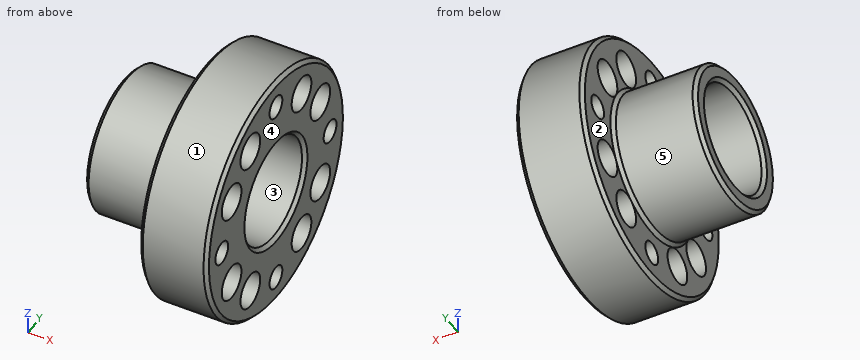
```python
from build123d import *

# Parameters (mm, degrees)
SKETCH2_R              = 3.25
CUT_EXTRUDE1_DEPTH     = 66.849562641
CHAMFER1_SIZE          = 1
SKETCH3_R              = 5
LIGHTENING_HOLES_DEPTH = 66.849562641


with BuildPart() as part:
    # Sketch1 → Revolve1 (revolve)
    with BuildSketch(Plane(origin=(0, 0, 0), x_dir=(1, 0, 0), z_dir=(0, 1, 0)), mode=Mode.PRIVATE) as revolve1_sk:
        Polygon((0, 20), (24, 20), (24, 35), (43.43, 35), (43.43, 15), (0, 15), align=None)
    revolve(revolve1_sk.sketch.rotate(Axis((0, 0, 0), (1, 0, 0)), 180), axis=Axis((0, 0, 0), (1, 0, 0)))

    # Sketch2 → Cut-Extrude1 (cut, through all)
    with BuildSketch(Plane(origin=(43.43, 0, 0), x_dir=(0, 0, -1), z_dir=(1, 0, 0))):
        with Locations((0, 27.5)):
            Circle(SKETCH2_R)
        with Locations((27.5, 0)):
            Circle(SKETCH2_R)
        with Locations((-27.5, 0)):
            Circle(SKETCH2_R)
        with Locations((0, -27.5)):
            Circle(SKETCH2_R)
    extrude(amount=-CUT_EXTRUDE1_DEPTH, mode=Mode.SUBTRACT)

    # Chamfer1
    chamfer1_edges = [part.edges().sort_by_distance(p)[0] for p in [
        (0, 0, -15),
        (43.43, 0, -15),
        (43.43, 0, -35),
        (24, 0, -35),
        (24, 0, -20),
        (0, 0, -20),
    ]]
    chamfer(chamfer1_edges, length=CHAMFER1_SIZE)

    # Sketch3 → lightening holes (cut, through all)
    with BuildSketch(Plane(origin=(43.43, 0, 0), x_dir=(0, 0, -1), z_dir=(1, 0, 0))):
        with Locations((13, 22.516660498)):
            Circle(SKETCH3_R)
        with Locations((22.516660498, 13)):
            Circle(SKETCH3_R)
        with Locations((22.516660498, -13)):
            Circle(SKETCH3_R)
        with Locations((13, -22.516660498)):
            Circle(SKETCH3_R)
        with Locations((-13, -22.516660498)):
            Circle(SKETCH3_R)
        with Locations((-22.516660498, -13)):
            Circle(SKETCH3_R)
        with Locations((-22.516660498, 13)):
            Circle(SKETCH3_R)
        with Locations((-13, 22.516660498)):
            Circle(SKETCH3_R)
    extrude(amount=-LIGHTENING_HOLES_DEPTH, mode=Mode.SUBTRACT)


solid = part.part
```
Here's how the part is built. I have some questions about the finished solid (model axes, mm). Face numbers are marked on the shaded views. A direction names the side the tool comes from. Give positions to 0.01 mm unless a question says otherwise; leave off trailing zeros. Loops run counter-clockwise (first coordinate to the right, second up) from the corner with the lowest first, then second, coordinate; pieces in that order, holes last. Notation, with made-up numbers: M 38.5,-35 L 66.5,-35 A20 ccw 66.5,-25 Z; hole C -23,84 d8. An arc over 180 degrees is marked long. Put each result on its own line as item: value. Start each with the question number.
(1) I want a section at D-D on x = 3. Please give me the cut outline in (y, z).
(2) Will these pins go through, and if not, where does the flat tip stop? pin 1 Ø7.5 at (y, z) = (27.5, 0) entering from -X; pin 2 Ø8 at (y, z) = (-13, -22.52) entering from +X; pin 3 Ø12 at (x, z) = (31, 15.5) entering from +Y; pin 4 Ø2 at (x, y) = (27.5, 11.5) entering from +Z.
(3) I need wall thicknesses on line 1 along Y through (x, z) = (35, -26); line 2 along Z through (x, y) = (41, -22.5); line 3 along Y through (x, z) = (27.5, 16.5). Which ranges of each line are inside material? Lowest first, please. Write a range as [from, to].
(4) For the marked faces 1 and 2, which set-ups out of +Z, -Z, +X, -X, +Y, -Y let a thin tool reach every point of the face, with its end or its side?
(5) I want a section at A-A on z = 0. State how many separate pieces and enclosed holes the cut face has, then the cut area to 3 significant figures.
(6) If we mould it in two halves opening along Z, with no side actions, what happens to the marked faces 3, 4 and 5? For each: +Z half, -Z half, draft (parallel to the pull), parting line (faces both ways), or undercut.
Answer block:
1. outline: C 0,0 d40; hole C 0,0 d30
2. pin 1: x = 24
2. pin 2: through
2. pin 3: y = 33.69
2. pin 4: z = 33.39
3. line 1: [-23.43, -16.59], [-9.41, -2.88], [2.88, 9.41], [16.59, 23.43]
3. line 2: [-26.81, -18], [-8, 8], [18, 26.81]
3. line 3: [-30.87, -26.09], [-18.95, 18.95], [26.09, 30.87]
4. face 1: +X, -X
4. face 2: -X
5. separate pieces: 4
5. enclosed holes: 0
5. area: 761 mm^2
6. face 3: undercut
6. face 4: draft
6. face 5: parting line
